from build123d import *

# Parameters (mm, degrees)
SKETCH1_R                = 2.97
SKETCH1_W                = 44.45
SKETCH1_H                = 2.2
BOSS_EXTRUDE1_DEPTH      = 44.45
CUT_EXTRUDE1_DEPTH       = 63.931914797
CUT_EXTRUDE1_DEPTH_BACK  = 63.931914797
SKETCH2_W                = 5.94
SKETCH2_H                = 17.78
FILLET1_R                = 6.35
SKETCH4_R                = 3.5
CUT_EXTRUDE2_DEPTH       = 63.931914797
F_5_16_CLEARANCE_HOLE1_D = 8.4328


with BuildPart() as part:
    # Sketch1 → Boss-Extrude1 (new, symmetric)
    with BuildSketch(Plane(origin=(0, 0, 0), x_dir=(1, 0, 0), z_dir=(0, 1, 0))):
        Circle(SKETCH1_R)
        with Locations((22.225, 1.1)):
            Rectangle(SKETCH1_W, SKETCH1_H)
    extrude(amount=BOSS_EXTRUDE1_DEPTH, both=True)

    # Sketch2 → Cut-Extrude1 (cut, two sides: drawn at the far end of the back side and taken through both)
    with BuildSketch(Plane.XY.offset(-CUT_EXTRUDE1_DEPTH_BACK)):
        with Locations((0, 35.56)):
            Rectangle(SKETCH2_W, SKETCH2_H)
        Rectangle(SKETCH2_W, SKETCH2_H)
        with Locations((0, -35.56)):
            Rectangle(SKETCH2_W, SKETCH2_H)
    extrude(amount=CUT_EXTRUDE1_DEPTH + CUT_EXTRUDE1_DEPTH_BACK, mode=Mode.SUBTRACT)

    # Fillet1
    fillet1_edges = [part.edges().sort_by_distance(p)[0] for p in [
        (44.45, 44.45, -1.1),
        (44.45, -44.45, -1.1),
    ]]
    fillet(fillet1_edges, radius=FILLET1_R)

    # Sketch4 → Cut-Extrude2 (cut, through all)
    with BuildSketch(Plane.XY):
        with Locations((27, 35.7)):
            Circle(SKETCH4_R)
        with Locations((27, -35.7)):
            Circle(SKETCH4_R)
    extrude(amount=-CUT_EXTRUDE2_DEPTH, mode=Mode.SUBTRACT)

    # 5/16 Clearance Hole1 (through all)
    with Locations(Plane.XY):
        with Locations((24.58125, 20.010345019), (24.58125, -20.010345019)):
            Hole(F_5_16_CLEARANCE_HOLE1_D / 2)


solid = part.part
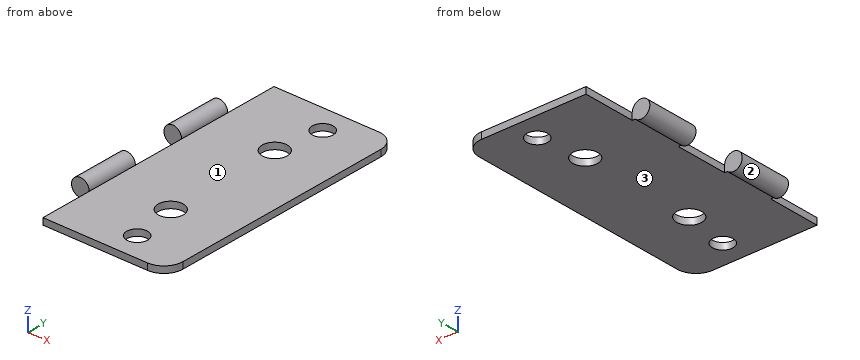
Verification items for the finished model (mm, model axes). Face numbers are marked on the shaded views. A direction names the side the tool comes from. Round coordinates to 2 decimals unless told otherwise and drop trailing zeros. Write each loop counter-clockwise with the first axis right and the second up, starting at its lowest first coordinate (ties: lowest second). Pieces come first, ordered by that corner, then holes.
(1) Section check B-B (x = 22.5). Enter the section's corners in (y, z).
Returned:
outline: (-44.45, -2.2) - (-23.68, -2.2) - (-23.68, 0) - (-44.45, 0) - close; (-16.34, -2.2) - (16.34, -2.2) - (16.34, 0) - (-16.34, 0) - close; (23.68, -2.2) - (44.45, -2.2) - (44.45, 0) - (23.68, 0) - close
(2) Section check A-A (y = -35.7). Enter the section's corners in (x, z).
Returned:
outline: (2.97, -2.2) - (23.5, -2.2) - (23.5, 0) - (2.97, 0) - close; (30.5, -2.2) - (44.45, -2.2) - (44.45, 0) - (30.5, 0) - close
(3) Section check D-D (y = -11.5). Enter the section's corners in (x, z).
Returned:
outline: (2, -2.2) - (44.45, -2.2) - (44.45, 0) - (2.97, 0) arc R2.97 ccw (long way) to start
(4) Section check C-C (z = -1). Enter the section's corners in (x, y), plus the area to 3 significant figures.
Returned:
outline: (-2.8, -26.67) - (2.97, -26.67) - (2.97, -44.45) - (38.1, -44.45) arc R6.35 ccw to (44.45, -38.1) - (44.45, 38.1) arc R6.35 ccw to (38.1, 44.45) - (2.97, 44.45) - (2.97, 26.67) - (-2.8, 26.67) - (-2.8, 8.89) - (2.97, 8.89) - (2.97, -8.89) - (-2.8, -8.89) - close; hole circle Ø8.43 at (24.58, -20.01); hole circle Ø8.43 at (24.58, 20.01); hole circle Ø7 at (27, -35.7); hole circle Ø7 at (27, 35.7)
area: 3,690 mm2
(5) Material ranges on line 1 (X direction, y = -36, z = -0.25); line 2 (Y direction, x = 27, z = -0.7); line 3 (Y direction, x = 1, z = -0.45), recorded low to high.
Returned:
line 1: x = 2.97 to 23.51, 30.49 to 44.45
line 2: y = -44.45 to -39.2, -32.2 to -23.46, -16.56 to 16.56, 23.46 to 32.2, 39.2 to 44.45
line 3: y = -26.67 to -8.89, 8.89 to 26.67
(6) Access from +Z, -Z, +X, -X, +Y, -Y to the whole of each face (thin tool, end or side, straight path). Record for the marked faces 1, 2 and 3.
Returned:
face 1: +Z, +X, +Y, -Y
face 2: +Y, -Y
face 3: -Z, +X, +Y, -Y
(7) Depth check by flat-ended pin: pin 1 Ø1 at (y, z) = (-4, 2) entering from +X; pin 2 Ø13.5 at (x, y) = (24.58, 20.01) entering from -Z; pin 3 Ø1.8 at (y, z) = (-0.5, -1) entering from -X; pin 4 Ø3 at (x, y) = (37.5, -24.5) entering from +Z. Enter the tip coordinate at first touch or a pass-through.
Returned:
pin 1: passes through
pin 2: stops at z = -2.2
pin 3: stops at x = 2.97
pin 4: stops at z = 0
